Geometry: final body of the model. Coordinates: model frame, mm. A direction names the side the tool comes from. Round coordinates to 2 decimals unless told otherwise and drop trailing zeros. Use CSV: the item, a comma, the result in double quotes.
from build123d import *

# Parameters (mm, degrees)
CORTE_EXTRUS_O1_REACH = 66.133
PADR_OCIRCULAR1_COUNT = 6


with BuildPart() as part:
    # Esboço5 → Revolução2 (revolve)
    with BuildSketch(Plane(origin=(0, 0, 0), x_dir=(1, 0, 0), z_dir=(0, 1, 0)), mode=Mode.PRIVATE) as revolu_o2_sk:
        with BuildLine():
            Line((30, 34.6), (30, 38))
            Line((30, 38), (35, 38))
            Line((35, 38), (35, 13.034480978))
            add(Edge.make_bspline(
                [(35, 13.034480978), (38.108675957, 10.648534591), (43.835508458, 9.861753235), (46.598549995, 10.040745389), (57.264939348, 12.650201836), (61, 12.65)],
                knots=[0, 0, 0, 0, 0.39411742, 0.49411742, 1, 1, 1, 1], degree=3))
            Line((61, 12.65), (61, 9.65))
            add(Edge.make_bspline(
                [(0, 28.6), (20.31391897, 8.95615601), (43.784583373, 4.835357072), (46.678252365, 5.00429716), (57.291609233, 9.661966126), (61, 9.65)],
                knots=[0, 0, 0, 0, 0.416422234, 0.516422234, 1, 1, 1, 1], degree=3))
            Line((0, 28.6), (0, 31.6))
            Line((0, 31.6), (3, 34.6))
            Line((3, 34.6), (30, 34.6))
        make_face()
    revolve(revolu_o2_sk.sketch.rotate(Axis((0, 0, 0), (1, 0, 0)), 180), axis=Axis((0, 0, 0), (1, 0, 0)))

    # Esboço30 → Corte-extrusão1 (cut, up to next)
    with BuildSketch(Plane(origin=(35, 0, 0), x_dir=(0, 0, -1), z_dir=(1, 0, 0)), mode=Mode.PRIVATE) as corte_extrus_o1_sk1:
        with BuildLine():
            Line((-14.798648587, 35), (14.798648587, 35))
            ThreePointArc((14.798648587, 35), (0, 38), (-14.798648587, 35))
        make_face()
    corte_extrus_o1_tool1 = extrude(corte_extrus_o1_sk1.sketch, amount=-CORTE_EXTRUS_O1_REACH, mode=Mode.PRIVATE) & part.part
    corte_extrus_o1 = corte_extrus_o1_tool1.solids().sort_by_distance((35, 36.204155, 0))[0]
    add(corte_extrus_o1, mode=Mode.SUBTRACT)

    # PadrãoCircular1: Corte-extrusão1 ×6 about axis
    padr_ocircular1_axis = Axis((0, 0, 0), (1, 0, 0))
    for i in range(1, PADR_OCIRCULAR1_COUNT):
        add(corte_extrus_o1.rotate(padr_ocircular1_axis, i * 360 / PADR_OCIRCULAR1_COUNT), mode=Mode.SUBTRACT)


solid = part.part
Item 1: Pin query (flat end, axial travel): P1, Ø8, axis at x = 14, y = 24.5, coming from the -Z side; P2, Ø5, axis at x = 40, z = -13.5, coming from the +Y side; P3, Ø5, axis at x = 34, z = -23, coming from the -Y side; P4, Ø2, axis at y = -24, z = 17, coming from the +X side. Return the tip coordinate at first contact, or that it passes through.
Final values:
P1,"stops at z = -27.87"
P2,"passes through"
P3,"stops at y = -32"
P4,"stops at x = 35"
Item 2: Reachability of faces 1 (the cylindrical face through (32.535, -32.942, -18.943)), 2 (the flat face through (35, -16, -1)), 3 (the cylindrical face through (16.7, -10.4, 33)) from +Z, -Z, +X, -X, +Y, -Y: full face, straight path, thin tool, end or side. Return the list, or none.
Final values:
face 1,"-Z, +X, -X, -Y"
face 2,"+X"
face 3,"-X"
Item 3: Material intervals for line 1 (X direction, y = -31, z = -4); line 2 (Y direction, x = 27, z = 7.5); line 3 (Y direction, x = 10, z = -2.5), sorted ascending.
Final values:
line 1,"x = 0 to 35"
line 2,"y = -33.78 to -6.66, 6.66 to 33.78"
line 3,"y = -34.51 to -19.91, 19.91 to 34.51"
